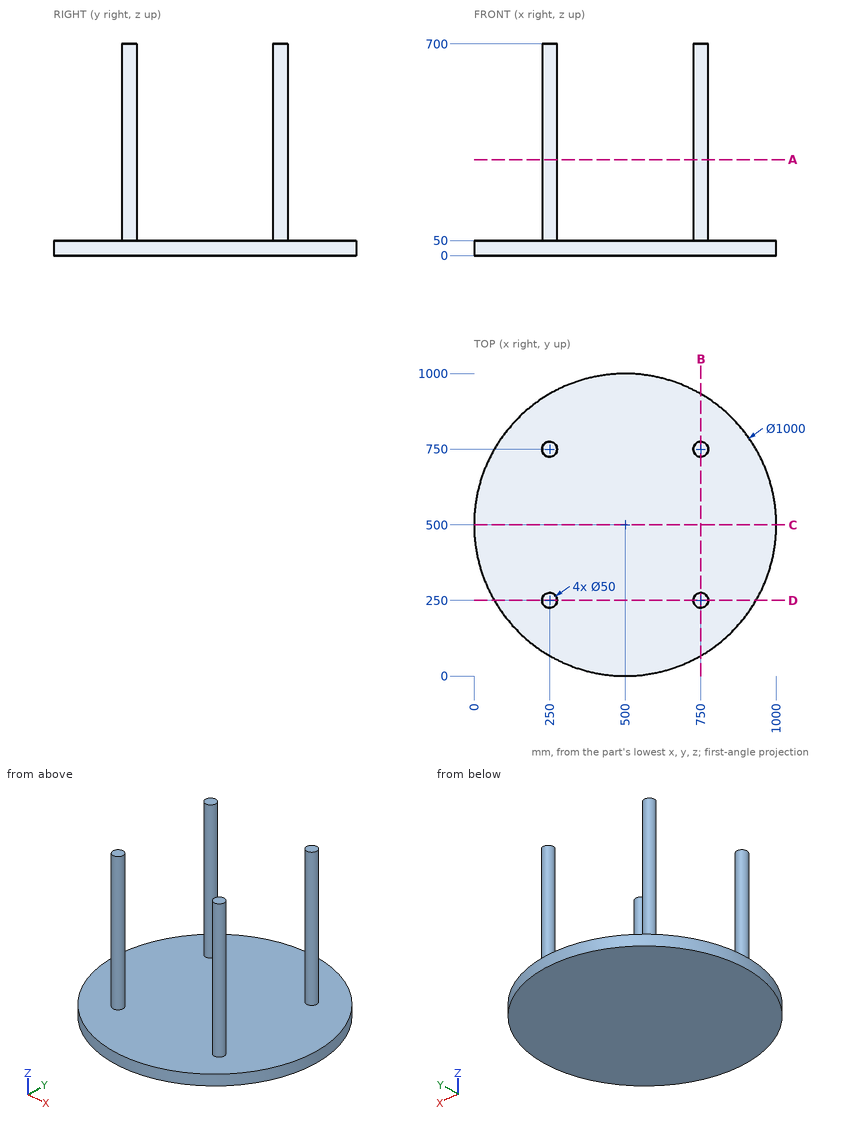
Geometry: see drawing. Coordinates: mm, zero at the bounding-box minimum. Round coordinates to 2 decimals unless told otherwise and drop trailing zeros. Write each loop counter-clockwise with the first axis right and the second up, starting at its lowest first coordinate (ties: lowest second). Pieces come first, ordered by that corner, then holes. Notation, with made-up numbers: (-19.5, 42.25) - (34.5, 42.25) arc R21 ccw to (34.5, 46.25) - close; hole circle Ø11 at (71.25, 40). An arc over 180 degrees is marked (long way). Use CSV: the item, a comma, the result in double quotes. Start each with the question number.
(1) First-contact query: pin 1 Ø4 at (x, y) = (804.5, 523.5) entering from +Z; pin 2 Ø12 at (x, y) = (309.5, 278.5) entering from -Z. Flat tips, straight axial feed; report the tip coordinate or a pass-through.
(2) Cut plane B-B, the plane x = 750. Return loops of the section in (y, z), and give its area (3 significant figures).
(3) Cut plane C-C, the plane y = 500. Return loops of the section in (x, z), and give its area (3 significant figures).
(4) Material intervals for probe 1 along Z at (x, y) = (396, 890); probe 2 along X at (y, z) = (249.5, 334) (3 decimals); probe 3 along Y at (x, z) = (262, 441.5), sorted ascending. Write a range as [from, to].
(5) Cut plane A-A, the plane z = 317.5. Return loops of the section in (x, y), and give its area (3 significant figures).
Geometry says:
1,pin 1,"z = 50"
1,pin 2,"z = 0"
2,outline,"(66.99, 0) - (933.01, 0) - (933.01, 50) - (775, 50) - (775, 700) - (725, 700) - (725, 50) - (275, 50) - (275, 700) - (225, 700) - (225, 50) - (66.99, 50) - close"
2,area,"108,000 mm²"
3,outline,"(0, 0) - (1000, 0) - (1000, 50) - (0, 50) - close"
3,area,"50,000 mm²"
4,probe 1,"[0, 50]"
4,probe 2,"[225.005, 274.995], [725.005, 774.995]"
4,probe 3,"[228.07, 271.93], [728.07, 771.93]"
5,outline,"circle Ø50 at (250, 250); circle Ø50 at (250, 750); circle Ø50 at (750, 250); circle Ø50 at (750, 750)"
5,area,"7,850 mm²"
